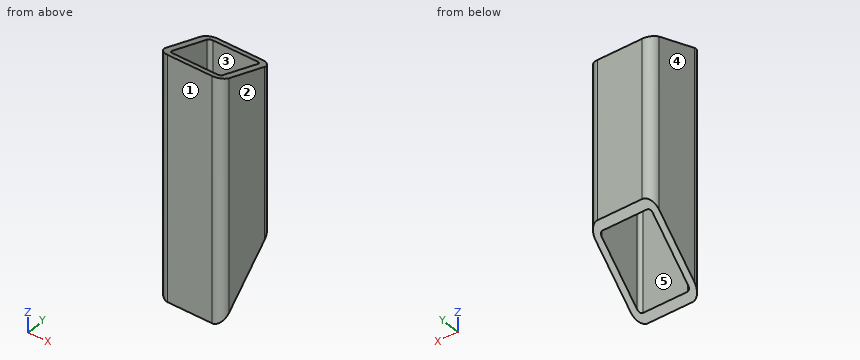
Autodesk Inventor part; units mm, degrees
ref_plane "Start Plane" through (0, 0, -10) normal (0, 0, 1) x (1, 0, 0)
ref_plane "End Plane" through (0, 0, 66.3002) normal (0, 0, 1) x (1, 0, 0)
ref_plane "Work Plane4" through (-7, -153.7024, 115.5399) normal (0, 0.3241, 0.946) x (1, 0, 0)
ref_plane "Start Plane" through (0, 0, -10) normal (0, 0, 1) x (1, 0, 0)
ref_plane "End Plane" through (0, 0, 66.3002) normal (0, 0, 1) x (1, 0, 0)
sketch "Sketch" plane through (0, 0, 0) normal (0, 0, 1) x (1, 0, 0)
  line L0 (-10, -7) -> (-10, 7)
  line L1 (-7, 10) -> (7, 10)
  line L2 (10, 7) -> (10, -7)
  line L3 (7, -10) -> (-7, -10)
  arc A0 (-10, -7) -> (-7, -10) centre (-7, -7) ccw
  arc A1 (-7, 10) -> (-10, 7) centre (-7, 7) ccw
  arc A2 (10, 7) -> (7, 10) centre (7, 7) ccw
  arc A3 (7, -10) -> (10, -7) centre (7, -7) ccw
  arc A4 (-7, 8) -> (-8, 7) centre (-7, 7) ccw
  line L4 (-7, 8) -> (7, 8)
  arc A5 (8, 7) -> (7, 8) centre (7, 7) ccw
  line L5 (8, 7) -> (8, -7)
  arc A6 (7, -8) -> (8, -7) centre (7, -7) ccw
  line L6 (7, -8) -> (-7, -8)
  arc A7 (-8, -7) -> (-7, -8) centre (-7, -7) ccw
  line L7 (-8, -7) -> (-8, 7)
  line L8 (0, 14.8698) -> (0, -14.8698) construction
  line L9 (-14.8698, 0) -> (14.8698, 0) construction
  dimension "d7" = 3
  dimension "d10" = 20
  dimension "d11" = 20
  dimension "d12" = 2
  dimension "d15" = 10
  dimension "d16" = 10
extrude "Body" add sketch "Sketch" along normal up to surface (76.3002 mm away) from surface at -10
sketch "Sketch3" plane through (0, 0, 0) normal (0, 0, 1) x (1, 0, 0)
  line L0 (0, 0) -> (10, 0)
ref_plane "Work Plane3" through (0, 0, 0) normal (0, -1, 0) x (1, 0, 0)
sketch "Sketch4" plane through (0, 0, 0) normal (0, -1, 0) x (1, 0, 0)
  line L0 (-2, -10) -> (12, -10)
  line L1 (-2, 66.3002) -> (12, 66.3002)
  dimension "d18" = 76.3002
ref_plane "Work Plane4" through (-7, -153.7024, 115.5399) normal (0, 0.3241, 0.946) x (1, 0, 0)
split "Split1" plane through (-7, -153.7024, 115.5399) removes the side toward (0, 0.3241, 0.946)
ref_plane "Work Plane7" through (0, -10, -10) normal (0, 0.7071, -0.7071) x (1, 0, 0)
split "Split4" plane through (0, -10, -10) removes the side toward (0, 0.7071, -0.7071)
equation "\"d7\" = G_IR"
equation "\"d10\" = G_H"
equation "\"d11\" = G_W"
equation "\"d12\" = G_T"
equation "\"d15\" = 0.5 * d10"
equation "\"d16\" = 0.5 * d11"
equation "\"d3\" = G_L"
equation "\"G_W\" = 20"
equation "\"G_H\" = 20"
equation "\"G_T\" = 2"
equation "\"G_IR\" = 3"
equation "\"G_L\" = d18"
equation "\"G_OFFSET_END\" = -7.14425"
equation "\"d14\" = G_OFFSET_END + B_L"
equation "\"B_L\" = 73.44444"
properties part number "ISO 12633-2 - 20x20x2 - 76,3" material "Steel, Mild"
Design review of the part built by this model. Coordinates are the model's own, in mm. Face numbers are marked on the shaded views. A direction names the side the tool comes from. Round coordinates to 2 decimals unless told otherwise and drop trailing zeros. Loops run counter-clockwise (first coordinate to the right, second up) from the corner with the lowest first, then second, coordinate; pieces in that order, holes last. Notation, with made-up numbers: (82, 78.5) - (115, 78.5) arc R8 ccw to (115, 88.5) - close; hole circle Ø4 at (64.5, -13.75). An arc over 180 degrees is marked (long way). One line per item, written item: value. Start each with the question number.
1) Consider section D-D on z = 4.5. Give the boundary of the cut face in (x, y).
2) For the marked faces 4 and 5, list the 3-axis set-ups (+Z, -Z, +X, -X, +Y, -Y) from which the entire face can be reached by the end or side of a thin tool; tool diameter is ignored.
3) Draft analysis for pull direction Y (two halves, no side actions). For the marked faces 1, 2 and 3, state which applies: +Y half, -Y half, draft (parallel to the pull), parting line (faces both ways), or undercut.
4) Consider section B-B on z = 24.5. Give the boundary of the cut face in (x, y), then the cut area to 3 significant figures.
5) To check wall thickness, follow L1, parallel to Y at x = 0.75, z = 37.5; L2, parallel to Y at x = 2, z = -2. State the ranges of each line that lie inside material, in increasing order. Write a range as from..to.
6) Consider section C-C on y = -6. Give the boundary of the cut face in (x, z), then the cut area to 3 significant figures.
Reported:
1. outline: (-10, -7) arc R3 ccw to (-7, -10) - (7, -10) arc R3 ccw to (10, -7) - (10, 4.5) - (8, 4.5) - (8, -7) arc R1 cw to (7, -8) - (-7, -8) arc R1 cw to (-8, -7) - (-8, 4.5) - (-10, 4.5) - close
2. face 4: +Z, -Z, -X, +Y, -Y
2. face 5: +Z, -Z
3. face 1: -Y half
3. face 2: draft
3. face 3: undercut
4. outline: (-10, -7) arc R3 ccw to (-7, -10) - (7, -10) arc R3 ccw to (10, -7) - (10, 7) arc R3 ccw to (7, 10) - (-7, 10) arc R3 ccw to (-10, 7) - close; hole (-8, -7) arc R1 ccw to (-7, -8) - (7, -8) arc R1 ccw to (8, -7) - (8, 7) arc R1 ccw to (7, 8) - (-7, 8) arc R1 ccw to (-8, 7) - close
4. area: 137 mm^2
5. L1: y = -10..-8, 8..10
5. L2: y = -10..-8
6. outline: (-10, -6) - (-8, -6) - (-8, 64.94) - (-10, 64.94) - close; (8, -6) - (10, -6) - (10, 64.94) - (8, 64.94) - close
6. area: 284 mm^2
